from build123d import *

# Parameters (mm, degrees)
F1_DEPTH = 114.3


with BuildPart() as f1:
    # F0 (on Top) → F1 (new body)
    with BuildSketch(Plane.XY):
        with BuildLine():
            Line((0, 0), (152.38726, 1.970525))
            Line((152.38726, 1.970525), (152.22305, 14.669463))
            Line((152.22305, 14.669463), (114.126235, 14.176832))
            Line((114.126235, 14.176832), (112.935709, 106.244135))
            Line((112.935709, 106.244135), (105.82064, 106.15213))
            ThreePointArc((105.82064, 106.15213), (105.822583, 105.951821), (105.82323, 105.751504))
            ThreePointArc((105.82323, 105.751504), (75.039211, 74.767815), (43.857148, 105.350878))
            Line((43.857148, 105.350878), (36.742079, 105.258873))
            Line((36.742079, 105.258873), (37.932605, 13.19157))
            Line((37.932605, 13.19157), (-0.16421, 12.698938))
            Line((-0.16421, 12.698938), (0, 0))
        make_face()
    extrude(amount=F1_DEPTH)


solid = f1.part
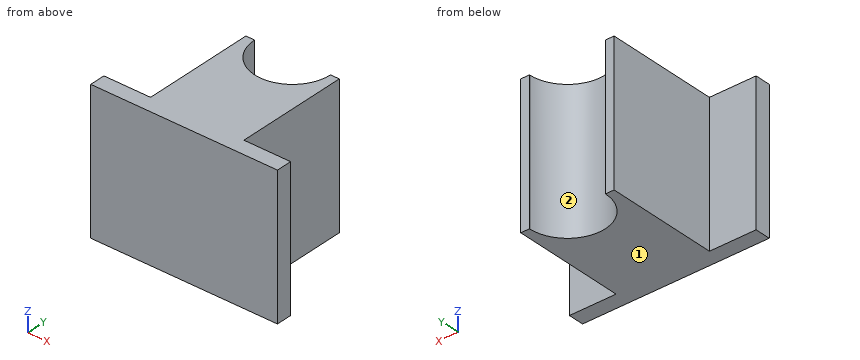
Geometry check sheet. Reference: the model listing, model coordinates, mm. Face numbers are marked on the shaded views. Coordinates: 2 decimals unless noted, no trailing zeros. Order: outer loops, then holes, each group sorted by start corner. A loop starts at its lowest first (then second) coordinate and runs counter-clockwise, first axis right, second up. Notation, with made-up numbers: (-14, 8) - (12, 8) arc R28 cw to (12, 42) - close; hole circle Ø4 at (36.25, 82). An arc over 180 degrees is marked (long way). Answer in a Markdown table with one row per item. Add a question column.
1) Release check for a two-part mould opening along X. For the marked faces 1 and 2 record: +X half, -X half, draft (parallel to the pull), parting line (faces both ways), or undercut.
2) Gauge pin test, flat ends, axial feed: P1, Ø1, axis at x = 88, z = 74, coming from the +Y side; P2, Ø1.5, axis at x = 122.5, z = 15.5, coming from the -Y side; P3, Ø12, axis at x = 92, z = 44, coming from the +Y side. Record the tip position at first contact, or that the pin passes through.
3) Material ranges on line 1 along X through (y, z) = (79, 29); line 2 along Y through (x, z) = (110, 76); line 3 along X through (y, z) = (32, 91), recorded low to high. Write a range as [from, to].
4) Cross-section at B-B, the plane z = 16.5. Record the cut outline in (x, y).
5) Cross-section at A-A, the plane y = 90. Record the cut outline in (x, z), then the cut area to 3 significant figures.
6) Cross-section at C-C, the plane x = 102. Record the cut outline in (y, z).
7) Cross-section at D-D, the plane y = 66. Record the cut outline in (x, z), then the cut area to 3 significant figures.
Check result:
| question | item | result |
|---|---|---|
| 1 | face 1 | draft |
| 1 | face 2 | undercut |
| 2 | P1 | stops at y = 77.94 |
| 2 | P2 | stops at y = 1.57 |
| 2 | P3 | stops at y = 85.17 |
| 3 | line 1 | x = [37.08, 59.21], [90.47, 113.29] |
| 3 | line 2 | y = [1.42, 106.21] |
| 3 | line 3 | x = [37.69, 113.9] |
| 4 | outline | (-0.16, 12.7) - (0, 0) - (152.39, 1.97) - (152.22, 14.67) - (114.13, 14.18) - (112.94, 106.24) - (105.82, 106.15) arc R30.96 cw to (105.82, 105.75) arc R30.98 cw to (43.86, 105.35) - (36.74, 105.26) - (37.93, 13.19) - close |
| 5 | outline | (36.94, 0) - (48.16, 0) - (48.16, 114.3) - (36.94, 114.3) - close; (101.52, 0) - (113.15, 0) - (113.15, 114.3) - (101.52, 114.3) - close |
| 5 | area | 2,610 mm² |
| 6 | outline | (1.32, 0) - (90.84, 0) - (90.84, 114.3) - (1.32, 114.3) - close |
| 7 | outline | (37.25, 0) - (113.46, 0) - (113.46, 114.3) - (37.25, 114.3) - close |
| 7 | area | 8,710 mm² |
